```python
from build123d import *

# Parameters (mm, degrees)
SKETCH1_W            = 108
SKETCH1_H            = 102
BOSS_EXTRUDE1_DEPTH  = 2
SKETCH2_W            = 104
SKETCH2_H            = 98
BOSS_EXTRUDE2_DEPTH  = 7
SKETCH3_W            = 100
SKETCH3_H            = 94
CUT_EXTRUDE1_DEPTH   = 7
SKETCH4_W            = 10
SKETCH4_H            = 3
BOSS_EXTRUDE6_DEPTH  = 1
CUT_EXTRUDE2_DEPTH   = 10
SKETCH6_W            = 10
SKETCH6_H            = 3
BOSS_EXTRUDE7_DEPTH  = 1
CUT_EXTRUDE3_DEPTH   = 10
SKETCH9_W            = 10
SKETCH9_H            = 3
BOSS_EXTRUDE9_DEPTH  = 1
CUT_EXTRUDE4_DEPTH   = 10
SKETCH11_W           = 10
SKETCH11_H           = 3
BOSS_EXTRUDE10_DEPTH = 1
CUT_EXTRUDE5_DEPTH   = 10
SKETCH20_W           = 10
SKETCH20_H           = 2
CUT_EXTRUDE7_DEPTH   = 2
SKETCH21_W           = 10
SKETCH21_H           = 2
CUT_EXTRUDE8_DEPTH   = 2
SKETCH22_W           = 10
SKETCH22_H           = 2
CUT_EXTRUDE9_DEPTH   = 2
SKETCH23_W           = 10
SKETCH23_H           = 2
CUT_EXTRUDE11_DEPTH  = 2
SKETCH24_R           = 2
BOSS_EXTRUDE11_DEPTH = 4
BOSS_EXTRUDE12_DEPTH = 4
BOSS_EXTRUDE13_DEPTH = 4
BOSS_EXTRUDE14_DEPTH = 4
SKETCH28_W           = 30
SKETCH28_H           = 2
BOSS_EXTRUDE15_DEPTH = 10
SKETCH29_R           = 2
SKETCH29_W           = 6
SKETCH29_H           = 4
CUT_EXTRUDE12_DEPTH  = 2
FILLET1_R            = 10
SKETCH30_W           = 30
SKETCH30_H           = 1
BOSS_EXTRUDE16_DEPTH = 10
CUT_EXTRUDE13_DEPTH  = 2
FILLET2_R            = 10


with BuildPart() as part:
    # Sketch1 → Boss-Extrude1 (new body)
    with BuildSketch(Plane(origin=(0, 0, 0), x_dir=(1, 0, 0), z_dir=(0, 1, 0))):
        Rectangle(SKETCH1_W, SKETCH1_H)
    extrude(amount=BOSS_EXTRUDE1_DEPTH)

    # Sketch2 → Boss-Extrude2 (add)
    with BuildSketch(Plane(origin=(0, 2, 0), x_dir=(1, 0, 0), z_dir=(0, 1, 0))):
        Rectangle(SKETCH2_W, SKETCH2_H)
    extrude(amount=BOSS_EXTRUDE2_DEPTH)

    # Sketch3 → Cut-Extrude1 (cut)
    with BuildSketch(Plane(origin=(0, 9, 0), x_dir=(1, 0, 0), z_dir=(0, 1, 0))):
        Rectangle(SKETCH3_W, SKETCH3_H)
    extrude(amount=-CUT_EXTRUDE1_DEPTH, mode=Mode.SUBTRACT)

    # Sketch4 → Boss-Extrude6 (add)
    with BuildSketch(Plane.XY.offset(49)):
        with Locations((-32, 7.5)):
            Rectangle(SKETCH4_W, SKETCH4_H)
    extrude(amount=BOSS_EXTRUDE6_DEPTH)

    # Sketch5 → Cut-Extrude2 (cut)
    with BuildSketch(Plane(origin=(-27, 0, 0), x_dir=(0, 0, -1), z_dir=(1, 0, 0))):
        Polygon((-50, 6), (-49, 9), (-50, 9), align=None)
    extrude(amount=-CUT_EXTRUDE2_DEPTH, mode=Mode.SUBTRACT)

    # Sketch6 → Boss-Extrude7 (add)
    with BuildSketch(Plane.XY.offset(49)):
        with Locations((32, 7.5)):
            Rectangle(SKETCH6_W, SKETCH6_H)
    extrude(amount=BOSS_EXTRUDE7_DEPTH)

    # Sketch7 → Cut-Extrude3 (cut)
    with BuildSketch(Plane(origin=(37, 0, 0), x_dir=(0, 0, -1), z_dir=(1, 0, 0))):
        Polygon((-50, 6), (-49, 9), (-50, 9), align=None)
    extrude(amount=-CUT_EXTRUDE3_DEPTH, mode=Mode.SUBTRACT)

    # Sketch9 → Boss-Extrude9 (add)
    with BuildSketch(Plane(origin=(0, 0, -49), x_dir=(-1, 0, 0), z_dir=(0, 0, -1))):
        with Locations((-32, 7.5)):
            Rectangle(SKETCH9_W, SKETCH9_H)
    extrude(amount=BOSS_EXTRUDE9_DEPTH)

    # Sketch10 → Cut-Extrude4 (cut)
    with BuildSketch(Plane.ZY.offset(-27)):
        Polygon((-49, 9), (-50, 6), (-50, 9), align=None)
    extrude(amount=-CUT_EXTRUDE4_DEPTH, mode=Mode.SUBTRACT)

    # Sketch11 → Boss-Extrude10 (add)
    with BuildSketch(Plane(origin=(0, 0, -49), x_dir=(-1, 0, 0), z_dir=(0, 0, -1))):
        with Locations((32, 7.5)):
            Rectangle(SKETCH11_W, SKETCH11_H)
    extrude(amount=BOSS_EXTRUDE10_DEPTH)

    # Sketch12 → Cut-Extrude5 (cut)
    with BuildSketch(Plane.ZY.offset(37)):
        Polygon((-49, 9), (-50, 6), (-50, 9), align=None)
    extrude(amount=-CUT_EXTRUDE5_DEPTH, mode=Mode.SUBTRACT)

    # Sketch20 → Cut-Extrude7 (cut)
    with BuildSketch(Plane.XY.offset(51)):
        with Locations((32, 1)):
            Rectangle(SKETCH20_W, SKETCH20_H)
    extrude(amount=-CUT_EXTRUDE7_DEPTH, mode=Mode.SUBTRACT)

    # Sketch21 → Cut-Extrude8 (cut)
    with BuildSketch(Plane(origin=(0, 2, 0), x_dir=(1, 0, 0), z_dir=(0, 1, 0))):
        with Locations((-32, -50)):
            Rectangle(SKETCH21_W, SKETCH21_H)
    extrude(amount=-CUT_EXTRUDE8_DEPTH, mode=Mode.SUBTRACT)

    # Sketch22 → Cut-Extrude9 (cut)
    with BuildSketch(Plane(origin=(0, 2, 0), x_dir=(1, 0, 0), z_dir=(0, 1, 0))):
        with Locations((32, 50)):
            Rectangle(SKETCH22_W, SKETCH22_H)
    extrude(amount=-CUT_EXTRUDE9_DEPTH, mode=Mode.SUBTRACT)

    # Sketch23 → Cut-Extrude11 (cut)
    with BuildSketch(Plane(origin=(0, 2, 0), x_dir=(1, 0, 0), z_dir=(0, 1, 0))):
        with Locations((-32, 50)):
            Rectangle(SKETCH23_W, SKETCH23_H)
    extrude(amount=-CUT_EXTRUDE11_DEPTH, mode=Mode.SUBTRACT)

    # Sketch24 → Boss-Extrude11 (add)
    with BuildSketch(Plane(origin=(0, 2, 0), x_dir=(1, 0, 0), z_dir=(0, 1, 0))):
        with Locations(Location((47, 44, 0), (0, 0, 270))):
            Circle(SKETCH24_R)
    extrude(amount=BOSS_EXTRUDE11_DEPTH)

    # Sketch25 → Boss-Extrude12 (add)
    with BuildSketch(Plane(origin=(0, 2, 0), x_dir=(1, 0, 0), z_dir=(0, 1, 0))):
        with BuildLine():
            ThreePointArc((-45, 44), (-45.585786438, 45.414213562), (-47, 46))
            Line((-47, 46), (-47, 44))
            Line((-47, 44), (-49, 44))
            ThreePointArc((-49, 44), (-47, 42), (-45, 44))
        make_face()
        with BuildLine():
            Line((-47, 44), (-47, 46))
            ThreePointArc((-47, 46), (-48.414213562, 45.414213562), (-49, 44))
            Line((-49, 44), (-47, 44))
        make_face()
    extrude(amount=BOSS_EXTRUDE12_DEPTH)

    # Sketch26 → Boss-Extrude13 (add)
    with BuildSketch(Plane(origin=(0, 2, 0), x_dir=(1, 0, 0), z_dir=(0, 1, 0))):
        with BuildLine():
            ThreePointArc((-49, -44), (-48.414213562, -45.414213562), (-47, -46))
            Line((-47, -46), (-47, -44))
            Line((-47, -44), (-49, -44))
        make_face()
        with BuildLine():
            Line((-47, -44), (-47, -46))
            ThreePointArc((-47, -46), (-45.585786438, -45.414213562), (-45, -44))
            ThreePointArc((-45, -44), (-47, -42), (-49, -44))
            Line((-49, -44), (-47, -44))
        make_face()
    extrude(amount=BOSS_EXTRUDE13_DEPTH)

    # Sketch27 → Boss-Extrude14 (add)
    with BuildSketch(Plane(origin=(0, 2, 0), x_dir=(1, 0, 0), z_dir=(0, 1, 0))):
        with BuildLine():
            ThreePointArc((49, -44), (45.585786438, -42.585786438), (47, -46))
            Line((47, -46), (47, -44))
            Line((47, -44), (49, -44))
        make_face()
        with BuildLine():
            Line((47, -44), (47, -46))
            ThreePointArc((47, -46), (48.414213562, -45.414213562), (49, -44))
            Line((49, -44), (47, -44))
        make_face()
    extrude(amount=BOSS_EXTRUDE14_DEPTH)

    # Sketch28 → Boss-Extrude15 (add)
    with BuildSketch(Plane.ZY.offset(54)):
        with Locations((0, 1)):
            Rectangle(SKETCH28_W, SKETCH28_H)
    extrude(amount=BOSS_EXTRUDE15_DEPTH)

    # Sketch29 → Cut-Extrude12 (cut)
    with BuildSketch(Plane(origin=(0, 2, 0), x_dir=(1, 0, 0), z_dir=(0, 1, 0))):
        with Locations((-58, 0)):
            Circle(SKETCH29_R)
        with Locations((-61, 0)):
            Rectangle(SKETCH29_W, SKETCH29_H)
    extrude(amount=-CUT_EXTRUDE12_DEPTH, mode=Mode.SUBTRACT)

    # Fillet1
    fillet1_edges = [part.edges().sort_by_distance(p)[0] for p in [
        (-64, 1, 15),
        (-64, 1, -15),
    ]]
    fillet(fillet1_edges, radius=FILLET1_R - 0.0001)  # a hair under: the kernel refuses the full size

    # Sketch30 → Boss-Extrude16 (add)
    with BuildSketch(Plane(origin=(54, 0, 0), x_dir=(0, 0, -1), z_dir=(1, 0, 0))):
        with Locations((0, 1.5)):
            Rectangle(SKETCH30_W, SKETCH30_H)
        with Locations((0, 0.5)):
            Rectangle(SKETCH30_W, SKETCH30_H)
    extrude(amount=BOSS_EXTRUDE16_DEPTH)

    # Sketch32 → Cut-Extrude13 (cut)
    with BuildSketch(Plane(origin=(0, 2, 0), x_dir=(1, 0, 0), z_dir=(0, 1, 0))):
        with BuildLine():
            Line((58, -2), (64, -2))
            Line((64, -2), (64, 2))
            Line((64, 2), (58, 2))
            ThreePointArc((58, 2), (59.414213562, 1.414213562), (60, 0))
            ThreePointArc((60, 0), (59.414213562, -1.414213562), (58, -2))
        make_face()
        with BuildLine():
            ThreePointArc((58, 2), (56, 0), (58, -2))
            Line((58, -2), (58, 2))
        make_face()
        with BuildLine():
            Line((58, 2), (58, -2))
            ThreePointArc((58, -2), (59.414213562, -1.414213562), (60, 0))
            ThreePointArc((60, 0), (59.414213562, 1.414213562), (58, 2))
        make_face()
    extrude(amount=-CUT_EXTRUDE13_DEPTH, mode=Mode.SUBTRACT)

    # Fillet2
    fillet2_edges = [part.edges().sort_by_distance(p)[0] for p in [
        (64, 1, -15),
        (64, 1, 15),
    ]]
    fillet(fillet2_edges, radius=FILLET2_R - 0.0001)  # a hair under: the kernel refuses the full size


solid = part.part
```
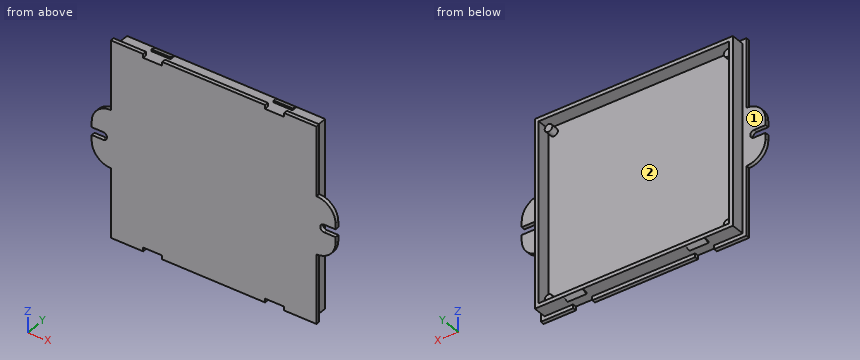
CAD build for the part. Positions are in the model's coordinates, mm. Face numbers are marked on the shaded views. Round coordinates to 2 decimals unless told otherwise and drop trailing zeros. Order: outer loops, then holes, each group sorted by start corner. A loop starts at its lowest first (then second) coordinate and runs counter-clockwise, first axis right, second up. Notation, with made-up numbers: (-8.75, 88) - (33.25, 88) arc R32 cw to (33.25, 123) - close; hole circle Ø7 at (45.5, -17). An arc over 180 degrees is marked (long way). Answer in a Markdown table with one row per item. Add a question column.
(1) Probe L1, parallel to Z at x = 49.5, y = 3.75; L2, parallel to X at y = 5.25, z = 14; L3, parallel to Y at x = 28.5, z = -17.5. List the from-to ranges inside material, lowest first. Write a range as [from, to].
(2) Band-saw the part on A-A on y = 3.5. List the corners of the cut face in (x, z), and give its area (3 significant figures).
(3) Band-saw the part on C-C on z = -40. List the corners of the cut face in (x, y).
(4) Band-saw the part on B-B on x = -14. List the corners of the cut face in (y, z), and give its area (3 significant figures).
(5) Drop flat-ended pins along their axis: pin 1 Ø1 at (x, z) = (16, -28.5) entering from +Y; pin 2 Ø1.6 at (y, z) = (1.5, -40.5) entering from +X; pin 3 Ø1 at (x, y) = (-60.5, 0.5) entering from -Z. Give the stop position or say it passes through.
(6) Mould opens along X. For the marked faces 1 and 2 say: +X half, -X half, draft (parallel to the pull), parting line (faces both ways), or undercut.
Data:
| question | item | result |
|---|---|---|
| 1 | L1 | z = [-49, -47], [47, 49] |
| 1 | L2 | x = [-52, -50], [50, 52] |
| 1 | L3 | y = [0, 2] |
| 2 | outline | (-52, -49) - (52, -49) - (52, 49) - (-52, 49) - close; circle Ø4 at (-47, -44); circle Ø4 at (-47, 44); circle Ø4 at (47, -44); circle Ø4 at (47, 44); hole (-50, -47) - (50, -47) - (50, 47) - (-50, 47) - close |
| 2 | area | 842 mm^2 |
| 3 | outline | (-54, 0) - (54, 0) - (54, 2) - (52, 2) - (52, 9) - (50, 9) - (50, 2) - (-50, 2) - (-50, 9) - (-52, 9) - (-52, 2) - (-54, 2) - close |
| 4 | outline | (0, -51) - (2, -51) - (2, -49) - (9, -49) - (9, -47) - (2, -47) - (2, 47) - (9, 47) - (9, 49) - (2, 49) - (2, 51) - (0, 51) - close |
| 4 | area | 232 mm^2 |
| 5 | pin 1 | stops at y = 2 |
| 5 | pin 2 | stops at x = 54 |
| 5 | pin 3 | stops at z = -13 |
| 6 | face 1 | draft |
| 6 | face 2 | undercut |
